Here's the drawing with two shaded views (mm, measured from the low corner). I have some questions. A direction names the side the tool comes from. Give positions to 0.01 mm unless a question says otherwise; leave off trailing zeros. Write each loop counter-clockwise with the first axis right and the second up, starting at its lowest first coordinate (ties: lowest second). Pieces come first, ordered by that corner, then holes. Notation, with made-up numbers: (0.25, -20.5) -> (55.25, -20.5) arc R16 ccw to (55.25, 3.5) -> close; hole circle Ø5 at (55.25, 23). An arc over 180 degrees is marked (long way). One line per item, written item: value.
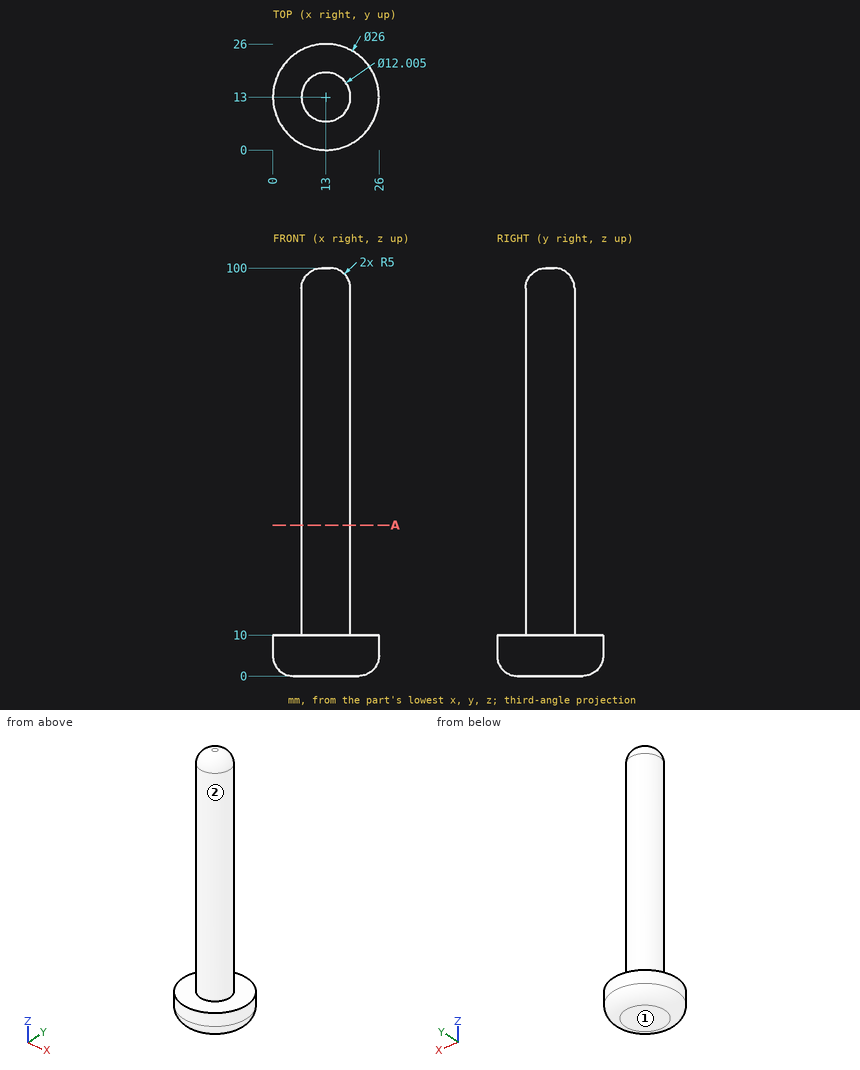
1) Will these pins go through, and if not, where does the flat tip stop? pin 1 (3 mm diameter, centred on x = 22.5, z = 66.5, fed in from +Y); pin 2 (6 mm diameter, centred on x = 12, y = 8, fed in from +Z); pin 3 (4 mm diameter, centred on y = 8, z = 21, fed in from +X); pin 4 (6 mm diameter, centred on y = 17.5, z = 16, fed in from -X).
Answer list:
pin 1: passes through
pin 2: stops at z = 99.88
pin 3: stops at x = 18.2
pin 4: stops at x = 7.19
2) For the marked faces 1 and 2, which set-ups out of +Z, -Z, +X, -X, +Y, -Y let a thin tool reach every point of the face, with its end or its side?
Answer list:
face 1: -Z, +X, -X, +Y, -Y
face 2: +Z
3) I need wall thicknesses on L1, parallel to Z at x = 10.5, y = 18.75; L2, parallel to Y at x = 13.25, z = 58. Which ranges of each line are inside material? Lowest first, please.
Answer list:
L1: z = 0 to 10
L2: y = 7 to 19
4) If we section it at A-A (z = 37): Write out the boundary of the cut face in (x, y) (1 decimal).
Answer list:
outline: circle Ø12 at (13, 13)
